Input: part model. Units: mm. Frame: model coordinates. Face numbers are marked on the shaded views. Coordinates: 2 decimals unless noted, no trailing zeros. Order: outer loops, then holes, each group sorted by start corner. A loop starts at its lowest first (then second) coordinate and runs counter-clockwise, first axis right, second up. Notation, with made-up numbers: (12.25, -22) -> (32.25, -22) arc R15 ccw to (32.25, -1) -> close; hole circle Ø1 at (-27, 30). An arc over 180 degrees is marked (long way). Write each question's results on one line, items separated by ' | '.
```python
from build123d import *

# Parameters (mm, degrees)
BOSS_EXTRUDE1_DEPTH            = 3.5
BOSS_EXTRUDE1_DEPTH_BACK       = 3.5
SKETCH2_R                      = 1.25
CUT_EXTRUDE1_DEPTH             = 3.5
BOSS_EXTRUDE2_START            = 0.5
SKETCH3_R                      = 2.25
SKETCH3_R_2                    = 1.25
BOSS_EXTRUDE2_DEPTH            = 0.5
CUT_EXTRUDE2_REACH             = 49.958
SKETCH4_R                      = 1.5
CUT_EXTRUDE2_DIRECTION_2_REACH = 49.958


with BuildPart() as part:
    # Sketch1 → Boss-Extrude1 (new, two sides: drawn at the far end of the back side and taken through both)
    with BuildSketch(Plane.XY.offset(-BOSS_EXTRUDE1_DEPTH_BACK)):
        Polygon((-46.3, 0), (46.3, 0), (46.3, -12), (44.8, -12), (44.8, -1.5), (-44.8, -1.5), (-44.8, -12), (-46.3, -12), align=None)
    extrude(amount=BOSS_EXTRUDE1_DEPTH + BOSS_EXTRUDE1_DEPTH_BACK)

    # Sketch2 → Cut-Extrude1 (cut)
    with BuildSketch(Plane(origin=(0, 0, 0), x_dir=(1, 0, 0), z_dir=(0, 1, 0))):
        with Locations(Location((0, 0, 0), (0, 0, 270))):
            Circle(SKETCH2_R)
    extrude(amount=-CUT_EXTRUDE1_DEPTH, mode=Mode.SUBTRACT)

    # Sketch3 → Boss-Extrude2 (add)
    with BuildSketch(Plane(origin=(0, 0, 0), x_dir=(1, 0, 0), z_dir=(0, 1, 0)).offset(BOSS_EXTRUDE2_START)):
        with Locations(Location((0, 0, 0), (0, 0, 270))):
            Circle(SKETCH3_R)
        with Locations(Location((0, 0, 0), (0, 0, 270))):
            Circle(SKETCH3_R_2, mode=Mode.SUBTRACT)
    extrude(amount=-BOSS_EXTRUDE2_DEPTH)

    # Cut-Extrude2: up to this face of the body (flat: up to its plane)
    cut_extrude2_end = Plane(part.part.faces().sort_by_distance((-46.3, -6, 0))[0])
    # Sketch4 → Cut-Extrude2 (cut, up to the picked face)
    with BuildSketch(Plane(origin=(0, 0, 0), x_dir=(0, 0, -1), z_dir=(1, 0, 0)), mode=Mode.PRIVATE) as cut_extrude2_sk1:
        with Locations((0, -8.5)):
            Circle(SKETCH4_R)
    cut_extrude2_tool1 = split(extrude(cut_extrude2_sk1.sketch, amount=-CUT_EXTRUDE2_REACH, mode=Mode.PRIVATE), bisect_by=cut_extrude2_end, keep=Keep.BOTH, mode=Mode.PRIVATE)
    add(cut_extrude2_tool1.solids().sort_by(Axis((0, -8.5, 0), (-1, 0, 0)))[0], mode=Mode.SUBTRACT)

    # Cut-Extrude2 direction 2: up to this face of the body (flat: up to its plane)
    cut_extrude2_direction_2_end = Plane(part.part.faces().sort_by_distance((46.3, -6, 0))[0])
    # Sketch4 → Cut-Extrude2 direction 2 (cut, up to the picked face)
    with BuildSketch(Plane(origin=(0, 0, 0), x_dir=(0, 0, -1), z_dir=(1, 0, 0)), mode=Mode.PRIVATE) as cut_extrude2_direction_2_sk1:
        with Locations((0, -8.5)):
            Circle(SKETCH4_R)
    cut_extrude2_direction_2_tool1 = split(extrude(cut_extrude2_direction_2_sk1.sketch, amount=CUT_EXTRUDE2_DIRECTION_2_REACH, mode=Mode.PRIVATE), bisect_by=cut_extrude2_direction_2_end, keep=Keep.BOTH, mode=Mode.PRIVATE)
    add(cut_extrude2_direction_2_tool1.solids().sort_by(Axis((0, -8.5, 0), (1, 0, 0)))[0], mode=Mode.SUBTRACT)


solid = part.part
```
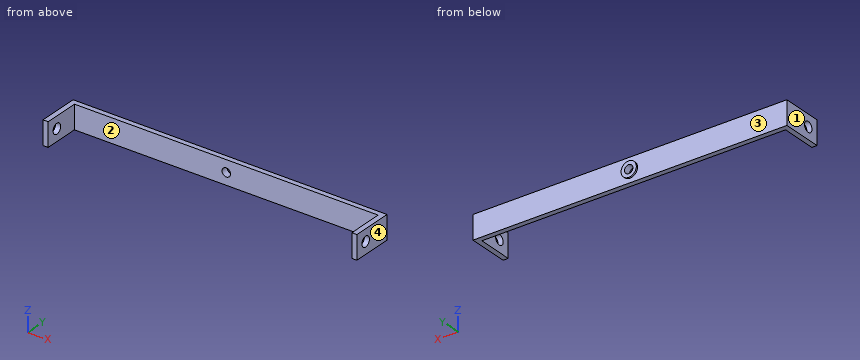
(1) Cut plane A-A, the plane y = -8.5. Return loops of the section in (x, z).
Return value:
outline: (-46.3, -3.5) -> (-44.8, -3.5) -> (-44.8, -1.5) -> (-46.3, -1.5) -> close; (-46.3, 1.5) -> (-44.8, 1.5) -> (-44.8, 3.5) -> (-46.3, 3.5) -> close; (44.8, -3.5) -> (46.3, -3.5) -> (46.3, -1.5) -> (44.8, -1.5) -> close; (44.8, 1.5) -> (46.3, 1.5) -> (46.3, 3.5) -> (44.8, 3.5) -> close
(2) Pin query (flat end, axial travel): P1, Ø2, axis at x = -18, z = -1.5, coming from the -Y side; P2, Ø2.5, axis at y = -8.5, z = 0, coming from the -X side. Return the tip coordinate at first contact, or that it passes through.
Return value:
P1: y = -1.5 | P2: through
(3) Cut plane C-C, the plane x = 0. Return loops of the section in (y, z), plus the area to 3 significant figures.
Return value:
outline: (-1.5, -3.5) -> (0, -3.5) -> (0, -2.25) -> (0.5, -2.25) -> (0.5, -1.25) -> (-1.5, -1.25) -> close; (-1.5, 1.25) -> (0.5, 1.25) -> (0.5, 2.25) -> (0, 2.25) -> (0, 3.5) -> (-1.5, 3.5) -> close | area: 7.75 mm2
(4) Cut plane B-B, the plane z = 0. Return loops of the section in (x, y).
Return value:
outline: (-46.3, -12) -> (-44.8, -12) -> (-44.8, -10) -> (-46.3, -10) -> close; (-46.3, -7) -> (-44.8, -7) -> (-44.8, -1.5) -> (-1.25, -1.5) -> (-1.25, 0.5) -> (-2.25, 0.5) -> (-2.25, 0) -> (-46.3, 0) -> close; (1.25, -1.5) -> (44.8, -1.5) -> (44.8, -7) -> (46.3, -7) -> (46.3, 0) -> (2.25, 0) -> (2.25, 0.5) -> (1.25, 0.5) -> close; (44.8, -12) -> (46.3, -12) -> (46.3, -10) -> (44.8, -10) -> close
(5) Cut plane D-D, the plane x = 23. Return loops of the section in (y, z).
Return value:
outline: (-1.5, -3.5) -> (0, -3.5) -> (0, 3.5) -> (-1.5, 3.5) -> close
(6) Mould query, pull axis X, two halves, no side actions, for the marked faces 1, 2, 3 and 4. Classes: +X half, -X half, draft (parallel to the pull), parting line (faces both ways), or undercut.
Return value:
face 1: -X half | face 2: undercut | face 3: draft | face 4: +X half
(7) Line query: line 1 along Z through (x, y) = (45.75, -8.5); line 2 along X through (y, z) = (-4.25, -2.5); line 3 along X through (y, z) = (-1, 0). Output: solid intervals per line, ascending. Write a range as from..to.
Return value:
line 1: -3.5..-1.5, 1.5..3.5 | line 2: -46.3..-44.8, 44.8..46.3 | line 3: -46.3..-1.25, 1.25..46.3
